Could you check a few things on this model? Use its own coordinates, in mm. Face numbers are marked on the shaded views. Give positions to 0.01 mm unless a question says otherwise; leave off trailing zeros. Loops run counter-clockwise (first coordinate to the right, second up) from the corner with the lowest first, then second, coordinate; pieces in that order, holes last. Notation, with made-up numbers: M -36,-2 L -14,-2 A23 cw -14,15 Z; hole C 11.25,-21.5 d11. An arc over 180 degrees is marked long. Answer in a Markdown table with one row per item. Add a question column.
1. I need wall thicknesses on line 1 along Z through (x, y) = (0, 7.5); line 2 along X through (y, z) = (17.5, 1); line 3 along Z through (x, y) = (1.6, 1.5). Which ranges of each line are inside material? Lowest first, please. Write a range as from..to.
2. Thinking about a two-plate mould opening in X: for the marked faces 1, 2 and 3, which applies, released by +X, released by -X, zero draft, split by the parting line, or undercut?
3. If we section it at A-A on x = 0: List the corners of the cut face in (y, z) for me, then the cut area to 3 significant figures.
4. If we section it at B-B on y = 9.25: List the corners of the cut face in (x, z) for me, then the cut area to 3 significant figures.
5. If we section it at C-C on z = 2: List the corners of the cut face in (x, y) for me, then the cut area to 3 significant figures.
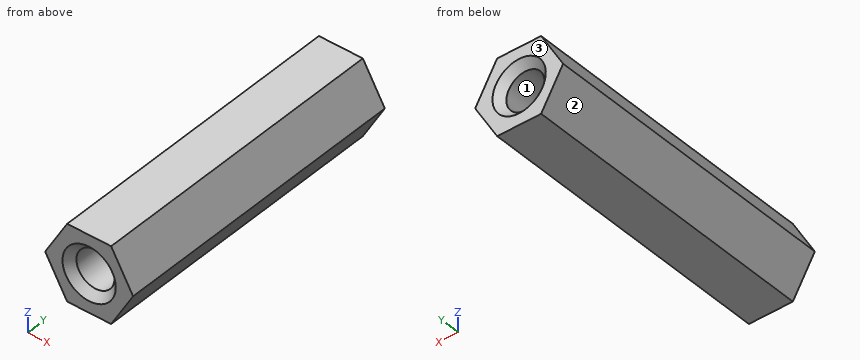
```python
from build123d import *

# Parameters (mm, degrees)
EXTRUDE_1_DEPTH = 20


with BuildPart() as part:
    # Эскиз1 → Бобышка-Вытянуть1 (new body)
    with BuildSketch(Plane(origin=(0, 0, 0), x_dir=(1, 0, 0), z_dir=(0, 1, 0))):
        Polygon((2.886751346, 0), (1.443375673, 2.5), (-1.443375673, 2.5), (-2.886751346, 0), (-1.443375673, -2.5), (1.443375673, -2.5), align=None)
    extrude(amount=EXTRUDE_1_DEPTH)

    # Эскиз2 → Отверстие обработанное метчиком M3x0.51 (revolve, cut)
    with BuildSketch(Plane(origin=(0, 20, 0), x_dir=(0, 0, 1), z_dir=(1, 0, 0))):
        Polygon((0, 0), (0, 20), (1.75, 20), (1.25, 19.5), (1.25, 0.5), (1.75, 0), align=None)
    revolve(axis=Axis((0, 26.35, 0), (0, -1, 0)), mode=Mode.SUBTRACT)


solid = part.part
```
Results:
| question | item | result |
|---|---|---|
| 1 | line 1 | -2.5..-1.25, 1.25..2.5 |
| 1 | line 2 | -2.31..-0.75, 0.75..2.31 |
| 1 | line 3 | -2.23..2.23 |
| 2 | face 1 | undercut |
| 2 | face 2 | released by -X |
| 2 | face 3 | zero draft |
| 3 | outline | M 0,-2.5 L 20,-2.5 L 20,-1.75 L 19.5,-1.25 L 0.5,-1.25 L 0,-1.75 Z; M 0,1.75 L 0.5,1.25 L 19.5,1.25 L 20,1.75 L 20,2.5 L 0,2.5 Z |
| 3 | area | 49.5 mm2 |
| 4 | outline | M -2.89,0 L -1.44,-2.5 L 1.44,-2.5 L 2.89,0 L 1.44,2.5 L -1.44,2.5 Z; hole C 0,0 d2.5 |
| 4 | area | 16.7 mm2 |
| 5 | outline | M -1.73,0 L 1.73,0 L 1.73,20 L -1.73,20 Z |
| 5 | area | 69.3 mm2 |
